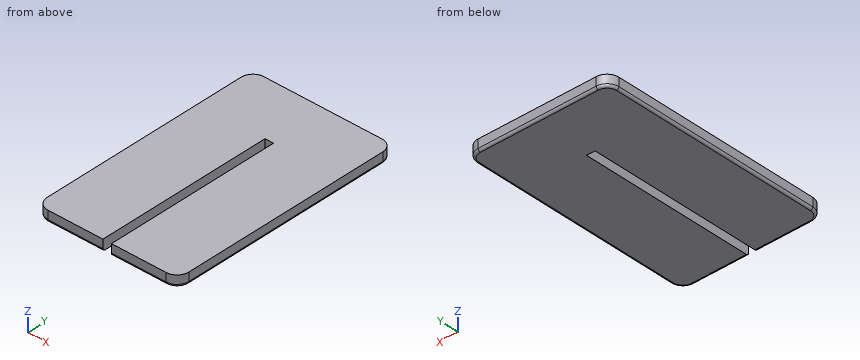
```python
from build123d import *

# Parameters (mm, degrees)
F1_DEPTH = 2.3
F2_R     = 2.5
F3_R     = 0.5


with BuildPart() as f1:
    # F0 (on Top) → F1 (new body)
    with BuildSketch(Plane.XY):
        Polygon((15, 24.75), (-15, 24.75), (-15, -24.75), (-0.9, -24.75), (-0.9, 12.45), (0.9, 12.45), (0.9, -24.75), (15, -24.75), align=None)
    extrude(amount=F1_DEPTH)

    # F2
    f2_edges = [f1.edges().sort_by_distance(p)[0] for p in [
        (-15, 24.75, 1.15),
        (-15, -24.75, 1.15),
        (15, -24.75, 1.15),
        (15, 24.75, 1.15),
    ]]
    fillet(f2_edges, radius=F2_R)

    # F3
    f3_edges = [f1.edges().sort_by_distance(p)[0] for p in [
        (6.7, -24.75, 0),
        (14.267767, -24.017767, 0),
        (15, 0, 0),
        (0, 24.75, 0),
        (14.267767, 24.017767, 0),
        (-14.267767, 24.017767, 0),
        (-15, 0, 0),
        (-14.267767, -24.017767, 0),
    ]]
    fillet(f3_edges, radius=F3_R)


solid = f1.part
```
Work out the finished part from the listing and answer in its coordinate system (mm). Round coordinates to 2 decimals unless told otherwise and drop trailing zeros. Write each loop counter-clockwise with the first axis right and the second up, starting at its lowest first coordinate (ties: lowest second). Pieces come first, ordered by that corner, then holes.
1) A cutting plane is placed at C-C on x = 0. Determine the outline of the cut face in (y, z), and give its area (3 significant figures).
2) A cutting plane is placed at B-B on z = 1.95. Determine the outline of the cut face in (x, y).
3) Consider probe 1 along X at (y, z) = (-5, 1.2); probe 2 along Y at (x, z) = (0.75, 1.1); probe 3 along Y at (x, z) = (-1.75, 0.4). Determine where each line is inside the solid, lowest interval first.
4) A cutting plane is placed at A-A on y = -18.5. Determine the outline of the cut face in (x, z).
Entries:
1. outline: (12.45, 0) - (24.25, 0) arc R0.5 ccw to (24.75, 0.5) - (24.75, 2.3) - (12.45, 2.3) - close
1. area: 28.2 mm2
2. outline: (-15, -22.25) arc R2.5 ccw to (-12.5, -24.75) - (-0.9, -24.75) - (-0.9, 12.45) - (0.9, 12.45) - (0.9, -24.75) - (12.5, -24.75) arc R2.5 ccw to (15, -22.25) - (15, 22.25) arc R2.5 ccw to (12.5, 24.75) - (-12.5, 24.75) arc R2.5 ccw to (-15, 22.25) - close
3. probe 1: x = -15 to -0.9, 0.9 to 15
3. probe 2: y = 12.45 to 24.75
3. probe 3: y = -24.74 to 24.74
4. outline: (-15, 0.5) arc R0.5 ccw to (-14.5, 0) - (-0.9, 0) - (-0.9, 2.3) - (-15, 2.3) - close; (0.9, 0) - (14.5, 0) arc R0.5 ccw to (15, 0.5) - (15, 2.3) - (0.9, 2.3) - close
